For this review, take the finished solid that the model builds, in its own axes (mm). Round coordinates to 2 decimals unless told otherwise and drop trailing zeros. Loops run counter-clockwise (first coordinate to the right, second up) from the corner with the lowest first, then second, coordinate; pieces in that order, holes last. Notation, with made-up numbers: (39, 84.25) -> (57, 84.25) arc R19 cw to (57, 108.25) -> close; hole circle Ø4 at (1.5, 40.5). An arc over 180 degrees is marked (long way). Write each question's results on one line, items separated by ' | '.
Autodesk Inventor part; units mm, degrees
ref_plane "YZ Plane" through (0, 0, 0) normal (1, 0, 0) x (0, 1, 0)
ref_plane "XZ Plane" through (0, 0, 0) normal (0, 1, 0) x (-1, 0, 0)
ref_plane "XY Plane" through (0, 0, 0) normal (0, 0, 1) x (1, 0, 0)
sketch "スケッチ1" plane through (0, 0, 0) normal (0, 0, 1) x (1, 0, 0)
  circle A0 centre (0, 0) radius 1.5
  circle A1 centre (15, 0) radius 1.5
  arc A2 (-0.8333, 4.9301) -> (-0.8333, -4.9301) centre (0, 0) ccw
  arc A3 (13.75, -7.3951) -> (13.75, 7.3951) centre (15, 0) ccw
  line L0 (-0.8333, 4.9301) -> (13.75, 7.3951)
  line L1 (-0.8333, -4.9301) -> (13.75, -7.3951)
  dimension "d0" = 3
  dimension "d1" = 3
  dimension "d2" = 15
  dimension "d3" = 10
  dimension "d4" = 15
extrude "押し出し1" add sketch "スケッチ1" along normal blind 3
properties part number "ウイング抑え" material "ポリカーボネート、クリア"
1. To check wall thickness, follow probe 1 along Y at (x, z) = (15, 0.7); probe 2 along X at (y, z) = (-0.5, 2.3); probe 3 along Y at (x, z) = (1, 1.75). State the ranges of each line that lie inside material, in increasing order.
Values found:
probe 1: y = -7.5 to -1.5, 1.5 to 7.5 | probe 2: x = -4.97 to -1.41, 1.41 to 13.59, 16.41 to 22.48 | probe 3: y = -5.24 to -1.12, 1.12 to 5.24
2. For pin 1 (1.5 mm diameter, centred on x = 19.5, z = 2, fed in from +Y); pin 2 (1 mm diameter, centred on x = 17.5, z = 1.5, fed in from +Y), all flat-tipped, find the tip position at first contact; note any pin that passes through.
Values found:
pin 1: stops at y = 6.5 | pin 2: stops at y = 7.23
3. Consider section C-C (z = 0.95). State the section outline as (x, y) points, plus the area to 3 significant figures.
Values found:
outline: (-0.83, -4.93) -> (13.75, -7.4) arc R7.5 ccw (long way) to (13.75, 7.4) -> (-0.83, 4.93) arc R5 ccw to start; hole circle Ø3 at (0, 0); hole circle Ø3 at (15, 0) | area: 304 mm2
4. Consider section D-D (x = 0). State the section outline as (y, z) points.
Values found:
outline: (-5.07, 0) -> (-1.5, 0) -> (-1.5, 3) -> (-5.07, 3) -> close; (1.5, 0) -> (5.07, 0) -> (5.07, 3) -> (1.5, 3) -> close
5. Consider section B-B (x = 15). State the section outline as (y, z) points.
Values found:
outline: (-7.5, 0) -> (-1.5, 0) -> (-1.5, 3) -> (-7.5, 3) -> close; (1.5, 0) -> (7.5, 0) -> (7.5, 3) -> (1.5, 3) -> close
6. Consider section A-A (y = 0). State the section outline as (x, z) points, plus the area to 3 significant figures.
Values found:
outline: (-5, 0) -> (-1.5, 0) -> (-1.5, 3) -> (-5, 3) -> close; (1.5, 0) -> (13.5, 0) -> (13.5, 3) -> (1.5, 3) -> close; (16.5, 0) -> (22.5, 0) -> (22.5, 3) -> (16.5, 3) -> close | area: 64.5 mm2
7. Draft analysis for pull direction X (two halves, no side actions). For faces 1 (the face through (9, 0, 3)), 2 (the face through (6.356, -6.145, 1.479)), 3 (the face through (-1.5, -0.07, 1.48)), 4 (the face through (13.5, -0.07, 1.48)), state which applies: released by +X, released by -X, zero draft, split by the parting line, or undercut.
Values found:
face 1: zero draft | face 2: released by -X | face 3: undercut | face 4: undercut
